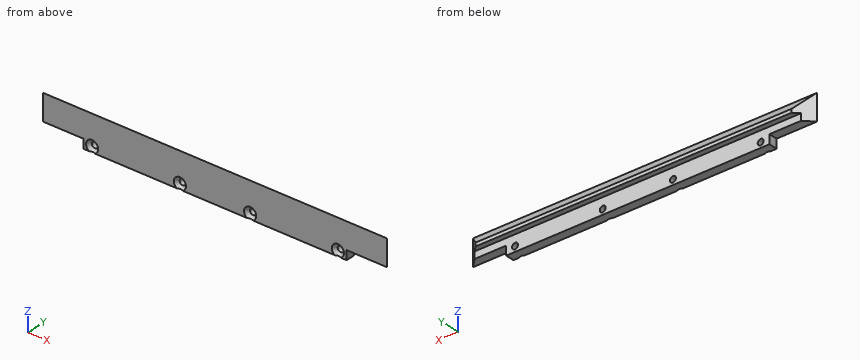
Autodesk Inventor part; units mm, degrees
ref_plane "YZ Plane" through (0, 0, 0) normal (1, 0, 0) x (0, 1, 0)
ref_plane "XZ Plane" through (0, 0, 0) normal (0, 1, 0) x (-1, 0, 0)
ref_plane "XY Plane" through (0, 0, 0) normal (0, 0, 1) x (1, 0, 0)
sketch "Szkic1" plane through (0, 0, 0) normal (1, 0, 0) x (0, 1, 0)
  line L0 (0, 0) -> (0, -20.1)
  line L1 (0, -20.1) -> (8, -20.1)
  line L2 (8, -20.1) -> (8, -9)
  line L3 (8, -9) -> (0, 0)
  line L4 (8, -20.1) -> (5, -20.1)
  line L5 (5, -20.1) -> (5, -11)
  line L6 (5, -11) -> (8, -11)
  line L7 (8, -11) -> (8, -20.1)
  line L8 (5, -14.9) -> (0, -14.9)
  dimension "d0" = 20.1
  dimension "d2" = 8
  dimension "d4" = 3
  dimension "d5" = 5.2
  dimension "d25" = 11
  dimension "d26" = 2
extrude "Wyciągnięcie proste1" add sketch "Szkic1" along normal mid plane 196 contours L3 L2 L6 L5 L8 L0
extrude "Wyciągnięcie proste2" add sketch "Szkic1" along normal mid plane 150 contours L8 L5 L1 L0
sketch "Szkic3" plane through (-98, 0, 0) normal (0, -1, 0) x (1, 0, 0)
  line L0 (98, 0) -> (98, -20.1) construction
  line L1 (23, -20.1) -> (173, -20.1) construction
  point P0 (168, -17.1)
  point P1 (118, -17.1)
  point P2 (28, -17.1)
  point P3 (78, -17.1)
  dimension "d12" = 20
  dimension "d13" = 70
  dimension "d14" = 3
hole "Otwór1" at (70, 0, -17.1) at (20, 0, -17.1) at (-20, 0, -17.1) at (-70, 0, -17.1) direction (0, 1, 0) diameter 3.4 end through all countersink diameter 6.9 countersink angle 84.225
sketch "Szkic4" plane through (75, 5, -20.1) normal (0, 0, -1) x (-1, 0, 0)
  line L0 (-23, 3) -> (-23, -5)
  line L1 (-23, -5) -> (-15, 3)
  line L2 (-23, 3) -> (173, 3) construction
  line L3 (-23, 3) -> (-23, -5)
  line L4 (-23, -5) -> (173, -5) construction
  line L5 (173, -5) -> (173, 3)
  line L6 (173, 3) -> (165, 3)
  line L7 (165, 3) -> (173, -5)
  line L8 (-23, 3) -> (-15, 3)
  point P0 (75, -5)
  dimension "d22" = 45
extrude "Wyciągnięcie proste3" cut sketch "Szkic4" against normal through all
properties part number "PlogPiramida"
For this review, take the finished solid that the model builds, in its own axes (mm). Round coordinates to 2 decimals unless told otherwise and drop trailing zeros. Order: outer loops, then holes, each group sorted by start corner. A loop starts at its lowest first (then second) coordinate and runs counter-clockwise, first axis right, second up. Notation, with made-up numbers: (48, 47) -> (90, 47) arc R21 cw to (90, 84) -> close; hole circle Ø5 at (0, 44.5). An arc over 180 degrees is marked (long way). Write item = value, one per line. Start each with the question number.
1) Take a section at C-C on x = -63. State the section outline as (y, z) points, plus the area to 3 significant figures.
2) Take a section at D-D on z = -4.75. State the section outline as (x, y) points, plus the area to 3 significant figures.
3) To check wall thickness, follow line 1 (X direction, y = 2.85, z = -17.1); line 2 (Z direction, x = 20, y = 4.35); line 3 (Y direction, x = -53, z = -13.5). State the ranges of each line that lie inside material, in increasing order. Write a range as from..to.
4) Take a section at A-A on x = -20. State the section outline as (y, z) points.
5) Insertion check: pin 1 (4 mm diameter, centred on x = -84.5, y = 2.5, fed in from -Z); pin 2 (2.5 mm diameter, centred on y = 1.5, z = -19, fed in from -X); pin 3 (3.5 mm diameter, centred on x = 6.5, y = 7, fed in from -Z); pin 4 (2 mm diameter, centred on x = -20, z = -17.1, fed in from -Y). Each pin has a flat end and moves straight along its axis. Give the tip position at first contact, or say it passes through.
6) Take a section at B-B on y = 3.5. State the section outline as (x, z) points.
Verdict:
q1.outline = (0, -20.1) -> (5, -20.1) -> (5, -11) -> (8, -11) -> (8, -9) -> (0, 0) -> close
q1.area = 97.5 mm2
q2.outline = (-98, 0) -> (98, 0) -> (93.78, 4.22) -> (-93.78, 4.22) -> close
q2.area = 810 mm2
q3.line_1 = -75..-71.7, -68.3..-21.7, -18.3..18.3, 21.7..68.3, 71.7..75
q3.line_2 = -20.1..-18.8, -15.4..-4.89
q3.line_3 = 0..5
q4.outline = (0, -13.65) -> (1.94, -15.4) -> (5, -15.4) -> (5, -11) -> (8, -11) -> (8, -9) -> (0, 0) -> close; (0.5, -20.1) -> (5, -20.1) -> (5, -18.8) -> (1.94, -18.8) -> close
q5.pin_1 = -14.9
q5.pin_2 = -75
q5.pin_3 = -11
q5.pin_4 = through
q6.outline = (-94.5, -14.9) -> (-75, -14.9) -> (-75, -20.1) -> (75, -20.1) -> (75, -14.9) -> (94.5, -14.9) -> (94.5, -3.94) -> (-94.5, -3.94) -> close; hole circle Ø3.4 at (-70, -17.1); hole circle Ø3.4 at (-20, -17.1); hole circle Ø3.4 at (20, -17.1); hole circle Ø3.4 at (70, -17.1)
